The drawing under review shows one solid part. Ordinate dimensions are in mm from its lowest x, y, z. A direction names the side the tool comes from. Coordinates: 2 decimals unless noted, no trailing zeros. Write each loop counter-clockwise with the first axis right and the second up, starting at its lowest first coordinate (ties: lowest second). Pieces come first, ordered by that corner, then holes.
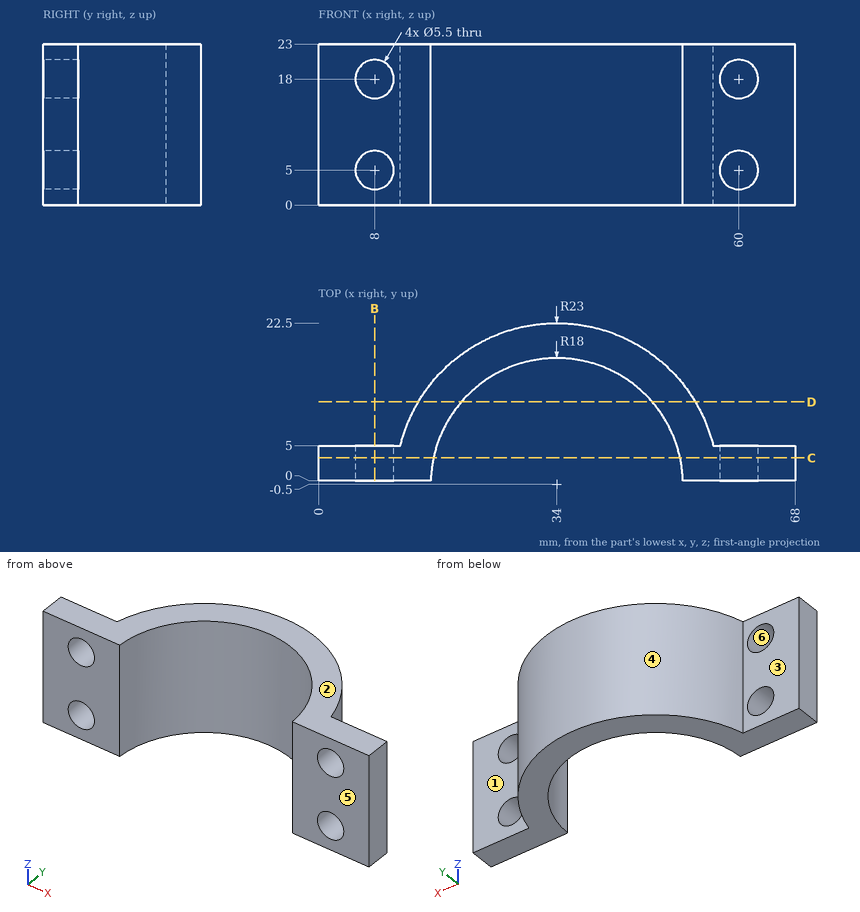
Q1. Draft analysis for pull direction X (two halves, no side actions). For the marked faces 4, 5 and 6, state which applies: +X half, -X half, draft (parallel to the pull), parting line (faces both ways), or undercut.
Ans:
face 4: parting line
face 5: draft
face 6: undercut
Q2. Add section B-B (x = 8). State the section outline as (y, z) points, then the cut area to 3 significant figures.
Ans:
outline: (0, 0) - (5, 0) - (5, 2.25) - (0, 2.25) - close; (0, 7.75) - (5, 7.75) - (5, 15.25) - (0, 15.25) - close; (0, 20.75) - (5, 20.75) - (5, 23) - (0, 23) - close
area: 60.0 mm2
Q3. For probe 1 along Z at (x, y) = (8, 3.8); probe 2 along Y at (x, z) = (50, 21.75); probe 3 along X at (y, z) = (3.75, 1), list the stretches that pass through material, from the lowest coordinate up.
Ans:
probe 1: z = 0 to 2.25, 7.75 to 15.25, 20.75 to 23
probe 2: y = 7.75 to 16.02
probe 3: x = 0 to 16.51, 51.49 to 68
Q4. Tool access review of the marked faces 1, 2 and 3: name each direction out of +Z, -Z, +X, -X, +Y, -Y from which nothing blocks a thin tool from reaching the whole face with its end or side.
Ans:
face 1: +Z, -Z, +X, +Y
face 2: +Z, +X, -X, +Y, -Y
face 3: +Z, -Z, -X, +Y
Q5. Clearance check with flat-ended pins moving along their axes: pin 1 Ø3.5 at (x, z) = (60, 18) entering from -Y; pin 2 Ø9 at (x, z) = (8, 5) entering from -Y; pin 3 Ø3.5 at (x, z) = (65, 17) entering from +Y; pin 4 Ø1 at (y, z) = (16.5, 5) entering from -X. State where each tip first meets the part, or that it passes through.
Ans:
pin 1: passes through
pin 2: stops at y = 0
pin 3: stops at y = 5
pin 4: stops at x = 17.98
Q6. Add section D-D (y = 11.25). State the section outline as (x, z) points, then the cut area to 3 significant figures.
Ans:
outline: (14.23, 0) - (20.36, 0) - (20.36, 23) - (14.23, 23) - close; (47.64, 0) - (53.77, 0) - (53.77, 23) - (47.64, 23) - close
area: 282 mm2
Q7. Add section C-C (y = 3.25). State the section outline as (x, z) points.
Ans:
outline: (0, 0) - (16.39, 0) - (16.39, 23) - (0, 23) - close; (51.61, 0) - (68, 0) - (68, 23) - (51.61, 23) - close; hole circle Ø5.5 at (8, 5); hole circle Ø5.5 at (8, 18); hole circle Ø5.5 at (60, 5); hole circle Ø5.5 at (60, 18)
